For this review, take the finished solid that the model builds, in its own axes (mm). Round coordinates to 2 decimals unless told otherwise and drop trailing zeros. Write each loop counter-clockwise with the first axis right and the second up, starting at its lowest first coordinate (ties: lowest second). Pieces come first, ordered by that corner, then holes.
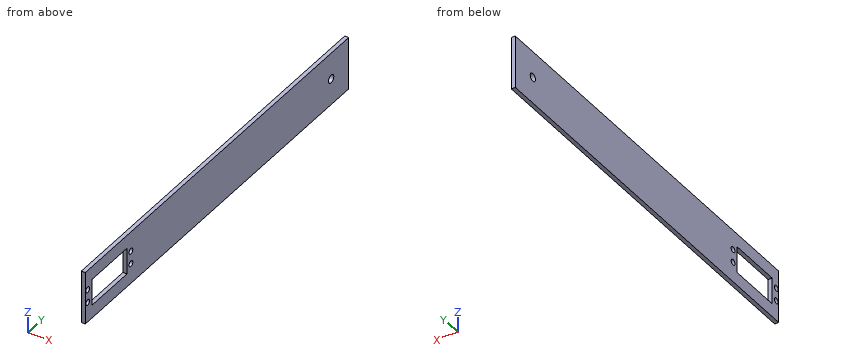
from build123d import *

# Parameters (mm, degrees)
SKETCH1_W           = 40
SKETCH1_H           = 300
BOSS_EXTRUDE1_DEPTH = 3
SKETCH2_R           = 3
CUT_EXTRUDE1_DEPTH  = 3
SKETCH3_R           = 2.15
SKETCH3_W           = 20
SKETCH3_H           = 40
CUT_EXTRUDE2_DEPTH  = 3


with BuildPart() as part:
    # Sketch1 → Boss-Extrude1 (new body)
    with BuildSketch(Plane(origin=(0, 0, 0), x_dir=(0, 0, -1), z_dir=(1, 0, 0))):
        Rectangle(SKETCH1_W, SKETCH1_H)
    extrude(amount=BOSS_EXTRUDE1_DEPTH)

    # Sketch2 → Cut-Extrude1 (cut)
    with BuildSketch(Plane(origin=(3, 0, 0), x_dir=(0, 0, -1), z_dir=(1, 0, 0))):
        with Locations((0, 130)):
            Circle(SKETCH2_R)
    extrude(amount=-CUT_EXTRUDE1_DEPTH, mode=Mode.SUBTRACT)

    # Sketch3 → Cut-Extrude2 (cut)
    with BuildSketch(Plane(origin=(3, 0, 0), x_dir=(0, 0, -1), z_dir=(1, 0, 0))):
        with Locations((-5.025, -147.31)):
            Circle(SKETCH3_R)
        with Locations((4.845, -147.31)):
            Circle(SKETCH3_R)
        with Locations((-5.025, -98.01)):
            Circle(SKETCH3_R)
        with Locations((4.845, -98.01)):
            Circle(SKETCH3_R)
        with Locations((0, -122.5)):
            Rectangle(SKETCH3_W, SKETCH3_H)
    extrude(amount=-CUT_EXTRUDE2_DEPTH, mode=Mode.SUBTRACT)


solid = part.part
(1) We need section D-D, the plane y = 130. Give the boundary of the cut face in (x, z), and give its area (3 significant figures).
Geometry check:
outline: (0, -20) - (3, -20) - (3, -3) - (0, -3) - close; (0, 3) - (3, 3) - (3, 20) - (0, 20) - close
area: 102 mm2
(2) For line 1 along Z through (x, y) = (2.25, -147.31) (3 decimals); line 2 along Y through (x, z) = (1.2, -9); line 3 along Y through (x, z) = (2.7, -0.5), list the stretches that pass through material, from the lowest coordinate up.
Geometry check:
line 1: z = -20 to -6.995, -2.695 to 2.875, 7.175 to 20
line 2: y = -150 to -142.5, -102.5 to 150
line 3: y = -150 to -142.5, -102.5 to 127.04, 132.96 to 150
(3) We need section B-B, the plane x = 1.1. Give the boundary of the cut face in (y, z) (3 decimals), and give its area (3 significant figures).
Geometry check:
outline: (-150, -20) - (150, -20) - (150, 20) - (-150, 20) - close; hole circle Ø4.3 at (-147.31, -4.845); hole circle Ø4.3 at (-147.31, 5.025); hole (-142.5, -10) - (-102.5, -10) - (-102.5, 10) - (-142.5, 10) - close; hole circle Ø4.3 at (-98.01, -4.845); hole circle Ø4.3 at (-98.01, 5.025); hole circle Ø6 at (130, 0)
area: 11,100 mm2
(4) We need section A-A, the plane y = -116. Give the boundary of the cut face in (x, z).
Geometry check:
outline: (0, -20) - (3, -20) - (3, -10) - (0, -10) - close; (0, 10) - (3, 10) - (3, 20) - (0, 20) - close
(5) We need section C-C, the plane z = 0. Give the boundary of the cut face in (x, y).
Geometry check:
outline: (0, -150) - (3, -150) - (3, -142.5) - (0, -142.5) - close; (0, -102.5) - (3, -102.5) - (3, 127) - (0, 127) - close; (0, 133) - (3, 133) - (3, 150) - (0, 150) - close
